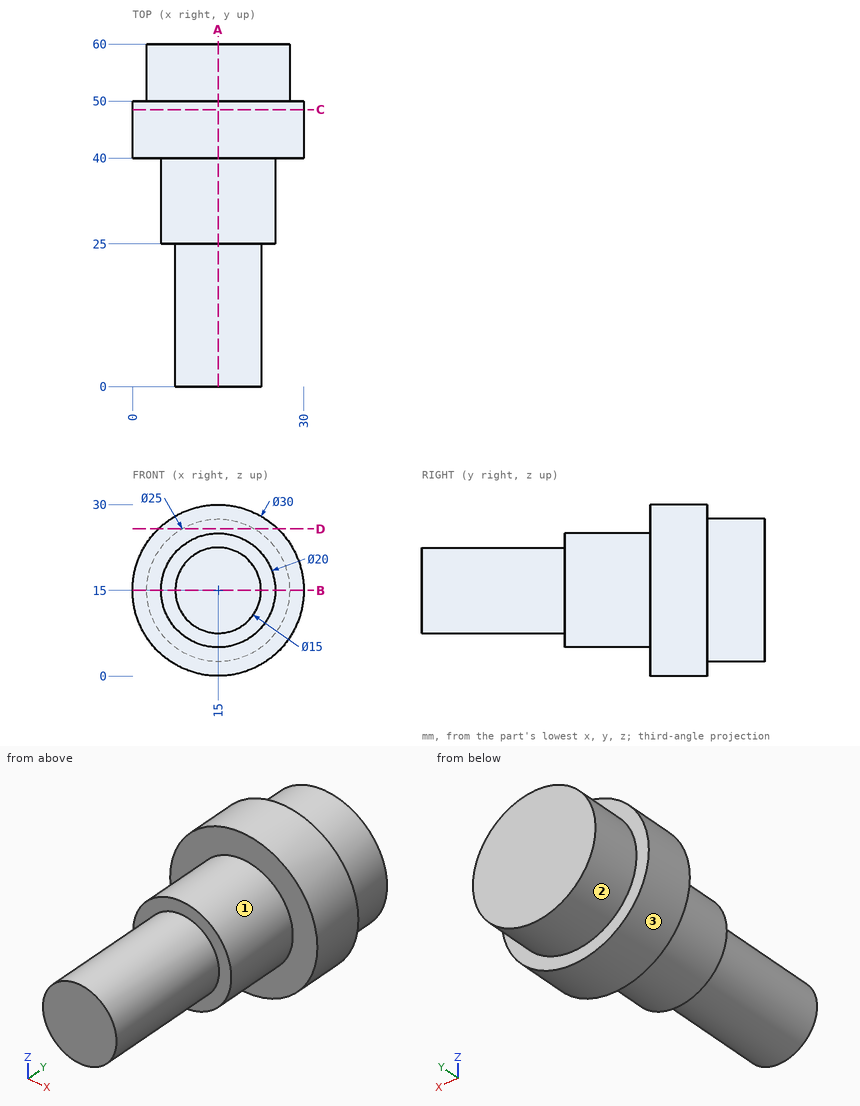
Answer from the drawing. Dimensions are ordinates in mm from the lowest x, y and z of the part. A direction names the side the tool comes from. Give positions to 0.01 mm unless a question says otherwise; leave off trailing zeros. Write each loop counter-clockwise with the first axis right and the second up, starting at its lowest first coordinate (ties: lowest second). Pieces come first, ordered by that corner, then holes. Notation, with made-up numbers: (2.5, 64) - (36.5, 64) arc R33 ccw to (36.5, 94) - close; hole circle Ø10 at (67.25, -28.5). An arc over 180 degrees is marked (long way). Answer in a Markdown table with one row per item. Add a question column.
Item 1: Find the intervals of material crossed by L1, parallel to X at y = 37, z = 15.5; L2, parallel to Y at x = 17, z = 2.5; L3, parallel to Y at x = 17.5, z = 24.75, in increasing order.
Item 2: Flat-ended cylindrical pins translate along their axes: P1, Ø3, axis at y = 7.5, z = 19.5, coming from the +X side; P2, Ø12, axis at x = 10, y = 33, coming from the -Z side; P3, Ø3, axis at x = 16.5, y = 31, coming from the +Z side. Find the tip coordinate at first contact, or state that the pin passes through.
Item 3: Section B-B, the plane z = 15 is taken. Write down the section's boundary in (x, y).
Item 4: Section D-D, the plane z = 25.75 is taken. Write down the section's boundary in (x, y).
Item 5: A tool of negligible diameter and unlimited length cuts with its end or side. For the marked faces 1, 2 and 3, from which of +Z, -Z, +X, -X, +Y, -Y can it reach the whole face along a straight path? Write none if from no direction.
Item 6: Section C-C, the plane y = 48.5 is taken. Write down the section's boundary in (x, z), and give its area (3 significant figures).
Item 7: Section A-A, the plane x = 15 is taken. Write down the section's boundary in (y, z), and give its area (4 significant figures).
Recorded:
| question | item | result |
|---|---|---|
| 1 | L1 | x = 5.01 to 24.99 |
| 1 | L2 | y = 40 to 50 |
| 1 | L3 | y = 40 to 60 |
| 2 | P1 | stops at x = 21.87 |
| 2 | P2 | stops at z = 5 |
| 2 | P3 | stops at z = 25 |
| 3 | outline | (0, 40) - (5, 40) - (5, 25) - (7.5, 25) - (7.5, 0) - (22.5, 0) - (22.5, 25) - (25, 25) - (25, 40) - (30, 40) - (30, 50) - (27.5, 50) - (27.5, 60) - (2.5, 60) - (2.5, 50) - (0, 50) - close |
| 4 | outline | (4.54, 40) - (25.46, 40) - (25.46, 50) - (21.38, 50) - (21.38, 60) - (8.62, 60) - (8.62, 50) - (4.54, 50) - close |
| 5 | face 1 | -Y |
| 5 | face 2 | +Y |
| 5 | face 3 | +Y, -Y |
| 6 | outline | circle Ø30 at (15, 15) |
| 6 | area | 707 mm2 |
| 7 | outline | (0, 7.5) - (25, 7.5) - (25, 5) - (40, 5) - (40, 0) - (50, 0) - (50, 2.5) - (60, 2.5) - (60, 27.5) - (50, 27.5) - (50, 30) - (40, 30) - (40, 25) - (25, 25) - (25, 22.5) - (0, 22.5) - close |
| 7 | area | 1,225 mm2 |
